```python
from build123d import *

# Parameters (mm, degrees)
CROQUIS1_R              = 29
SALIENTE_EXTRUIR1_DEPTH = 1
CROQUIS2_R              = 3
SALIENTE_EXTRUIR2_DEPTH = 7
SALIENTE_EXTRUIR3_START = -1
SALIENTE_EXTRUIR3_DEPTH = 1
CROQUIS4_R              = 3
SALIENTE_EXTRUIR4_DEPTH = 6
CROQUIS5_R              = 1.5
CORTAR_EXTRUIR1_DEPTH   = 6
CORTAR_EXTRUIR2_REACH   = 45.336
CROQUIS6_W              = 5.5
CROQUIS6_H              = 14.4
CROQUIS6_W_2            = 7.5
CROQUIS6_H_2            = 16


with BuildPart() as part:
    # Croquis1 → Saliente-Extruir1 (new body)
    with BuildSketch(Plane(origin=(0, 0, 0), x_dir=(1, 0, 0), z_dir=(0, 1, 0))):
        with Locations(Location((0, 0, 0), (0, 0, 270))):
            Circle(CROQUIS1_R)
    extrude(amount=SALIENTE_EXTRUIR1_DEPTH)

    # Croquis2 → Saliente-Extruir2 (add)
    with BuildSketch(Plane(origin=(0, 1, 0), x_dir=(1, 0, 0), z_dir=(0, 1, 0))):
        with Locations(Location((-15, 15, 0), (0, 0, 270))):
            Circle(CROQUIS2_R)
        with Locations(Location((15, 15, 0), (0, 0, 270))):
            Circle(CROQUIS2_R)
        with Locations(Location((-15, -15, 0), (0, 0, 270))):
            Circle(CROQUIS2_R)
        with Locations(Location((15, -15, 0), (0, 0, 270))):
            Circle(CROQUIS2_R)
    extrude(amount=SALIENTE_EXTRUIR2_DEPTH)

    # Croquis3 → Saliente-Extruir3 (add)
    with BuildSketch(Plane(origin=(0, 8, 0), x_dir=(1, 0, 0), z_dir=(0, 1, 0)).offset(SALIENTE_EXTRUIR3_START)):
        with BuildLine():
            Line((-15, -12), (-15, 12))
            ThreePointArc((-15, 12), (-12.878679656, 12.878679656), (-12, 15))
            Line((-12, 15), (12, 15))
            ThreePointArc((12, 15), (12.878679656, 12.878679656), (15, 12))
            Line((15, 12), (15, -12))
            ThreePointArc((15, -12), (12.878679656, -12.878679656), (12, -15))
            Line((12, -15), (-12, -15))
            ThreePointArc((-12, -15), (-12.878679656, -12.878679656), (-15, -12))
        make_face()
    extrude(amount=SALIENTE_EXTRUIR3_DEPTH)

    # Croquis4 → Saliente-Extruir4 (add)
    with BuildSketch(Plane(origin=(0, 8, 0), x_dir=(1, 0, 0), z_dir=(0, 1, 0))):
        with Locations(Location((15, 15, 0), (0, 0, 270))):
            Circle(CROQUIS4_R)
        with Locations(Location((15, -15, 0), (0, 0, 270))):
            Circle(CROQUIS4_R)
        with Locations(Location((-15, 15, 0), (0, 0, 270))):
            Circle(CROQUIS4_R)
        with Locations(Location((-15, -15, 0), (0, 0, 270))):
            Circle(CROQUIS4_R)
    extrude(amount=SALIENTE_EXTRUIR4_DEPTH)

    # Croquis5 → Cortar-Extruir1 (cut)
    with BuildSketch(Plane(origin=(0, 14, 0), x_dir=(1, 0, 0), z_dir=(0, 1, 0))):
        with Locations(Location((15, 15, 0), (0, 0, 270))):
            Circle(CROQUIS5_R)
        with Locations(Location((15, -15, 0), (0, 0, 270))):
            Circle(CROQUIS5_R)
        with Locations(Location((-15, -15, 0), (0, 0, 270))):
            Circle(CROQUIS5_R)
        with Locations(Location((-15, 15, 0), (0, 0, 270))):
            Circle(CROQUIS5_R)
    extrude(amount=-CORTAR_EXTRUIR1_DEPTH, mode=Mode.SUBTRACT)

    # Croquis6 → Cortar-Extruir2 (cut, up to next)
    with BuildSketch(Plane.XZ, mode=Mode.PRIVATE) as cortar_extruir2_sk1:
        with Locations((20, 0)):
            Rectangle(CROQUIS6_W, CROQUIS6_H)
    cortar_extruir2_tool1 = extrude(cortar_extruir2_sk1.sketch, amount=-CORTAR_EXTRUIR2_REACH, mode=Mode.PRIVATE) & part.part
    # Croquis6 → Cortar-Extruir2 (cut, up to next)
    with BuildSketch(Plane.XZ, mode=Mode.PRIVATE) as cortar_extruir2_sk2:
        with Locations((-20, 0)):
            Rectangle(CROQUIS6_W_2, CROQUIS6_H_2)
    cortar_extruir2_tool2 = extrude(cortar_extruir2_sk2.sketch, amount=-CORTAR_EXTRUIR2_REACH, mode=Mode.PRIVATE) & part.part
    add(cortar_extruir2_tool1.solids().sort_by_distance((20, 0, 0))[0], mode=Mode.SUBTRACT)
    add(cortar_extruir2_tool2.solids().sort_by_distance((-20, 0, 0))[0], mode=Mode.SUBTRACT)


solid = part.part
```
Verification items for the finished model (mm, model axes). A direction names the side the tool comes from. Round coordinates to 2 decimals unless told otherwise and drop trailing zeros. Write each loop counter-clockwise with the first axis right and the second up, starting at its lowest first coordinate (ties: lowest second). Pieces come first, ordered by that corner, then holes.
1. Section check D-D on y = 2.5. Enter the section's corners in (x, z).
2. Draft check along Y on faces 1 (the flat face through (0, 1, 0)), 2 (the cylindrical face through (-11.107, 0.493, 26.789)), 3 (the flat face through (0, 7, 0)), 4 (the flat face through (-16.3, 14, 16.3)). Enter one of: +Y half, -Y half, draft (parallel to the pull), parting line (faces both ways), or undercut.
3. Access from +Z, -Z, +X, -X, +Y, -Y to the whole of each face (thin tool, end or side, straight path). Record for faces 5 (the cylindrical face through (-14.93, 11.04, -16.5)), 6 (the flat face through (13.7, 14, 16.3)).
4. Section check B-B on y = 10.5. Enter the section's corners in (x, z), plus the area to 3 significant figures.
5. Section check C-C on z = 0. Enter the section's corners in (x, y), plus the area to 3 significant figures.
6. Scan lines: L1, parallel to X at y = 9.6, z = -15; L2, parallel to Y at x = -5.5, z = -4.5; L3, parallel to Y at x = 24.5, z = 1. Record each from-to range of solid material in increasing order.
7. Section check A-A on x = 0. Enter the section's corners in (y, z).
8. Gauge pin test, flat ends, axial feed: P1, Ø6, axis at x = 0.5, y = 9.5, coming from the +Z side; P2, Ø0.8, axis at y = 0.5, z = -3.5, coming from the +X side; P3, Ø2, axis at y = 3, z = -17, coming from the -X side. Record the tip position at first contact, or that the pin passes through.
Answer:
1. outline: circle Ø6 at (-15, -15); circle Ø6 at (-15, 15); circle Ø6 at (15, -15); circle Ø6 at (15, 15)
2. face 1: undercut
2. face 2: draft
2. face 3: undercut
2. face 4: +Y half
3. face 5: +Y
3. face 6: +Z, -Z, +X, -X, +Y
4. outline: circle Ø6 at (-15, -15); circle Ø6 at (-15, 15); circle Ø6 at (15, -15); circle Ø6 at (15, 15); hole circle Ø3 at (-15, -15); hole circle Ø3 at (-15, 15); hole circle Ø3 at (15, -15); hole circle Ø3 at (15, 15)
4. area: 84.8 mm2
5. outline: (-29, 0) - (-23.75, 0) - (-23.75, 1) - (-29, 1) - close; (-16.25, 0) - (17.25, 0) - (17.25, 1) - (-16.25, 1) - close; (-15, 7) - (15, 7) - (15, 8) - (-15, 8) - close; (22.75, 0) - (29, 0) - (29, 1) - (22.75, 1) - close
5. area: 75.0 mm2
6. L1: x = -18 to -16.5, -13.5 to -12, 12 to 13.5, 16.5 to 18
6. L2: y = 0 to 1, 7 to 8
6. L3: y = 0 to 1
7. outline: (0, -29) - (1, -29) - (1, 29) - (0, 29) - close; (7, -15) - (8, -15) - (8, 15) - (7, 15) - close
8. P1: stops at z = 15
8. P2: stops at x = 28.83
8. P3: stops at x = -17.83
